from build123d import *

# Parameters (mm, degrees)
BOSS_EXTRUDE1_DEPTH                      = 21
BOSS_EXTRUDE2_DEPTH                      = 10
CBORE_START                              = 17.5
CBORE_FOR_M5_HEX_HEAD_BOLT1_OUTLINE_R    = 6.119
CBORE_FOR_M5_HEX_HEAD_BOLT1_DEPTH        = 3.5
CBORE_START_2                            = 11.819091173
CBORE_FOR_M5_HEX_HEAD_BOLT1_2_OUTLINE_R  = 2.75
CBORE_FOR_M5_HEX_HEAD_BOLT1_2_DEPTH      = 5.680908827
CBORE_FOR_M10_HEX_HEAD_BOLT1_D           = 11
CBORE_FOR_M10_HEX_HEAD_BOLT1_CBORE_D     = 21.475
CBORE_FOR_M10_HEX_HEAD_BOLT1_CBORE_DEPTH = 6.4
F_4_0MM_DOWEL_HOLE1_D                    = 4
F_4_0MM_DOWEL_HOLE1_DEPTH                = 10
F_4_0MM_DOWEL_HOLE1_TIP                  = 1.201721238


# Read off the part's stored shape, not the designer's step: CBORE for M5 Hex Head Bolt1
with BuildPart() as part:
    # Sketch1 → Boss-Extrude1 (new body)
    with BuildSketch(Plane.XY):
        with BuildLine():
            Line((35, 65), (0, 65))
            Line((0, 65), (0, 0))
            Line((0, 0), (30, 0))
            ThreePointArc((30, 0), (75, 28.205505282), (120, 0))
            Line((120, 0), (155, 0))
            Line((155, 0), (155, 33.758563653))
            ThreePointArc((155, 33.758563653), (151.433820369, 47.944935308), (141.583123952, 58.758563653))
            Line((141.583123952, 58.758563653), (98.881926996, 87.083333333))
            ThreePointArc((98.881926996, 87.083333333), (96.317802362, 87.202818364), (95, 85))
            Line((95, 85), (95, 55))
            Line((95, 55), (75, 55))
            Line((75, 55), (75, 75))
            ThreePointArc((75, 75), (55, 95), (35, 75))
            Line((35, 75), (35, 65))
        make_face()
    extrude(amount=BOSS_EXTRUDE1_DEPTH)

    # Sketch2 → Boss-Extrude2 (add)
    with BuildSketch(Plane.XY):
        with BuildLine():
            Line((30, 0), (41.458980338, 0))
            ThreePointArc((41.458980338, 0), (75, 18.205505282), (108.541019662, 0))
            Line((108.541019662, 0), (120, 0))
            ThreePointArc((120, 0), (75, 28.205505282), (30, 0))
        make_face()
    extrude(amount=BOSS_EXTRUDE2_DEPTH)

    # Sketch16 → 1/16 Rc Tapped Hole1 (revolve, cut)
    with BuildSketch(Plane(origin=(8, 65, 10.5), x_dir=(0, 0, 1), z_dir=(1, 0, 0))):
        Polygon((0, 0), (0, 65), (3.05, 65), (3.05, 7.4), (3.339997004, 7.4), (3.571, 0), align=None)
    revolve(axis=Axis((8, 71.35, 10.5), (0, -1, 0)), mode=Mode.SUBTRACT)

    # CBORE for M5 Hex Head Bolt1 outline → CBORE for M5 Hex Head Bolt1 (cut)
    with BuildSketch(Plane.XY.offset(CBORE_START)):
        with Locations((8, 10)):
            Circle(CBORE_FOR_M5_HEX_HEAD_BOLT1_OUTLINE_R)
        with Locations((8, 25)):
            Circle(CBORE_FOR_M5_HEX_HEAD_BOLT1_OUTLINE_R)
        with Locations((8, 40)):
            Circle(CBORE_FOR_M5_HEX_HEAD_BOLT1_OUTLINE_R)
        with Locations((8, 55)):
            Circle(CBORE_FOR_M5_HEX_HEAD_BOLT1_OUTLINE_R)
    extrude(amount=CBORE_FOR_M5_HEX_HEAD_BOLT1_DEPTH, mode=Mode.SUBTRACT)

    # CBORE for M5 Hex Head Bolt1 2 outline → CBORE for M5 Hex Head Bolt1 2 (cut)
    with BuildSketch(Plane.XY.offset(CBORE_START_2)):
        with Locations((8, 10)):
            Circle(CBORE_FOR_M5_HEX_HEAD_BOLT1_2_OUTLINE_R)
        with Locations((8, 25)):
            Circle(CBORE_FOR_M5_HEX_HEAD_BOLT1_2_OUTLINE_R)
        with Locations((8, 40)):
            Circle(CBORE_FOR_M5_HEX_HEAD_BOLT1_2_OUTLINE_R)
        with Locations((8, 55)):
            Circle(CBORE_FOR_M5_HEX_HEAD_BOLT1_2_OUTLINE_R)
    extrude(amount=CBORE_FOR_M5_HEX_HEAD_BOLT1_2_DEPTH, mode=Mode.SUBTRACT)

    # CBORE for M10 Hex Head Bolt1 (through all)
    with Locations(Plane.XY.offset(21)):
        with Locations((28, 32.5), (55, 75), (140, 33.758563653)):
            CounterBoreHole(CBORE_FOR_M10_HEX_HEAD_BOLT1_D / 2, CBORE_FOR_M10_HEX_HEAD_BOLT1_CBORE_D / 2, CBORE_FOR_M10_HEX_HEAD_BOLT1_CBORE_DEPTH)

    # Ø4.0mm Dowel Hole1
    with Locations(Plane(origin=(70.328191882, 106.023738481, 0), x_dir=(0.8333333333333334, -0.5527707983925666, 0), z_dir=(0.5527707983925666, 0.8333333333333334, 0))):
        with Locations((42.264482137, -10.5)):
            Hole(F_4_0MM_DOWEL_HOLE1_D / 2, depth=F_4_0MM_DOWEL_HOLE1_DEPTH)
            with Locations((0, 0, -(F_4_0MM_DOWEL_HOLE1_DEPTH + F_4_0MM_DOWEL_HOLE1_TIP / 2))):  # 118° drill point
                Cone(0, F_4_0MM_DOWEL_HOLE1_D / 2, F_4_0MM_DOWEL_HOLE1_TIP, mode=Mode.SUBTRACT)


solid = part.part
Input: part model. Units: mm. Frame: model coordinates. A direction names the side the tool comes from. Give positions to 0.01 mm unless a question says otherwise; leave off trailing zeros. Loops run counter-clockwise (first coordinate to the right, second up) from the corner with the lowest first, then second, coordinate; pieces in that order, holes last. Notation, with made-up numbers: (-15.5, -35.75) -> (3.5, -35.75) arc R19 cw to (3.5, -18.75) -> close; hole circle Ø8 at (13, 82.5). An arc over 180 degrees is marked (long way). Answer as a JSON object with one key per item and string values. Group by question number.
Item 1: Cut plane D-D, the plane x = 113. Return the cut outline in (y, z), and give its area (3 significant figures).
Item 2: Cut plane B-B, the plane x = 28. Return the cut outline in (y, z).
Item 3: Line query: probe 1 along Y at (x, z) = (8, 18.3); probe 2 along Y at (x, z) = (28, 17.25); probe 3 along X at (y, z) = (10, 14.2). Output: solid intervals per line, ascending.
Item 4: Cut plane C-C, the plane x = 140. Return the cut outline in (y, z).
Item 5: Reachability of faces 4 (the conical face through (6.962, 61.352, 13.797)), 5 (the flat face through (95, 70, 10)), 6 (the cylindrical face through (10.54, 23.95, 15.25)), 7 (the flat face through (76, 38, 0)), 8 (the conical face through (99.242, 73.653, 10.711)) from +Z, -Z, +X, -X, +Y, -Y: full face, straight path, thin tool, end or side. Return the list, or none.
Item 6: Cut plane A-A, the plane z = 2.75. Return the cut outline in (x, y), and give its area (4 significant figures).
Item 7: Pin query (flat end, axial travel): P1, Ø3.5, axis at x = 8, y = 40, coming from the +Z side; P2, Ø6, axis at y = 72, z = 13, coming from the -X side; P3, Ø12, axis at x = 87.5, y = 14.5, coming from the +Z side. Return the tip coordinate at first contact, or that it passes through.
Item 8: Pull-direction query (X, two-part tool) for faces 1 (the flat face through (0, 33, 10)), 2 (the flat face through (76, 38, 21)), 3 (the cylindrical face through (137.672, 23.276, 17.845)); classes: released by +X, released by -X, zero draft, split by the parting line, or undercut.
Checks:
{
 "1": {"outline": "(0, 0) -> (77.72, 0) -> (77.72, 21) -> (10.7, 21) -> (10.7, 10) -> (0, 10) -> close", "area": "1,510 mm²"},
 "2": {"outline": "(0, 0) -> (27, 0) -> (27, 14.6) -> (21.76, 14.6) -> (21.76, 21) -> (0, 21) -> close; (38, 0) -> (65, 0) -> (65, 21) -> (43.24, 21) -> (43.24, 14.6) -> (38, 14.6) -> close"},
 "3": {"probe 1": "y = 0 to 3.88, 16.12 to 18.88, 31.12 to 33.88, 46.12 to 48.88, 61.12 to 65", "probe 2": "y = 0 to 21.76, 43.24 to 65", "probe 3": "x = 0 to 5.25, 10.75 to 36.41, 113.59 to 155"},
 "4": {"outline": "(0, 0) -> (28.26, 0) -> (28.26, 14.6) -> (23.02, 14.6) -> (23.02, 21) -> (0, 21) -> close; (39.26, 0) -> (59.81, 0) -> (59.81, 21) -> (44.5, 21) -> (44.5, 14.6) -> (39.26, 14.6) -> close"},
 "5": {"face 4": "+Y", "face 5": "+Z, -Z, +Y", "face 6": "+Z", "face 7": "-Z, +X, -X, +Y, -Y", "face 8": "none"},
 "6": {"outline": "(0, 0) -> (41.46, 0) arc R40 cw to (108.54, 0) -> (155, 0) -> (155, 33.76) arc R30 ccw to (141.58, 58.76) -> (98.88, 87.08) arc R2.5 ccw to (95, 85) -> (95, 55) -> (75, 55) -> (75, 75) arc R20 ccw to (35, 75) -> (35, 65) -> (0, 65) -> close; hole circle Ø11 at (28, 32.5); hole circle Ø11 at (55, 75); hole circle Ø11 at (140, 33.76)", "area": "10,000 mm²"},
 "7": {"P1": "stops at z = 8", "P2": "stops at x = 35", "P3": "stops at z = 10"},
 "8": {"face 1": "released by -X", "face 2": "zero draft", "face 3": "undercut"}
}
